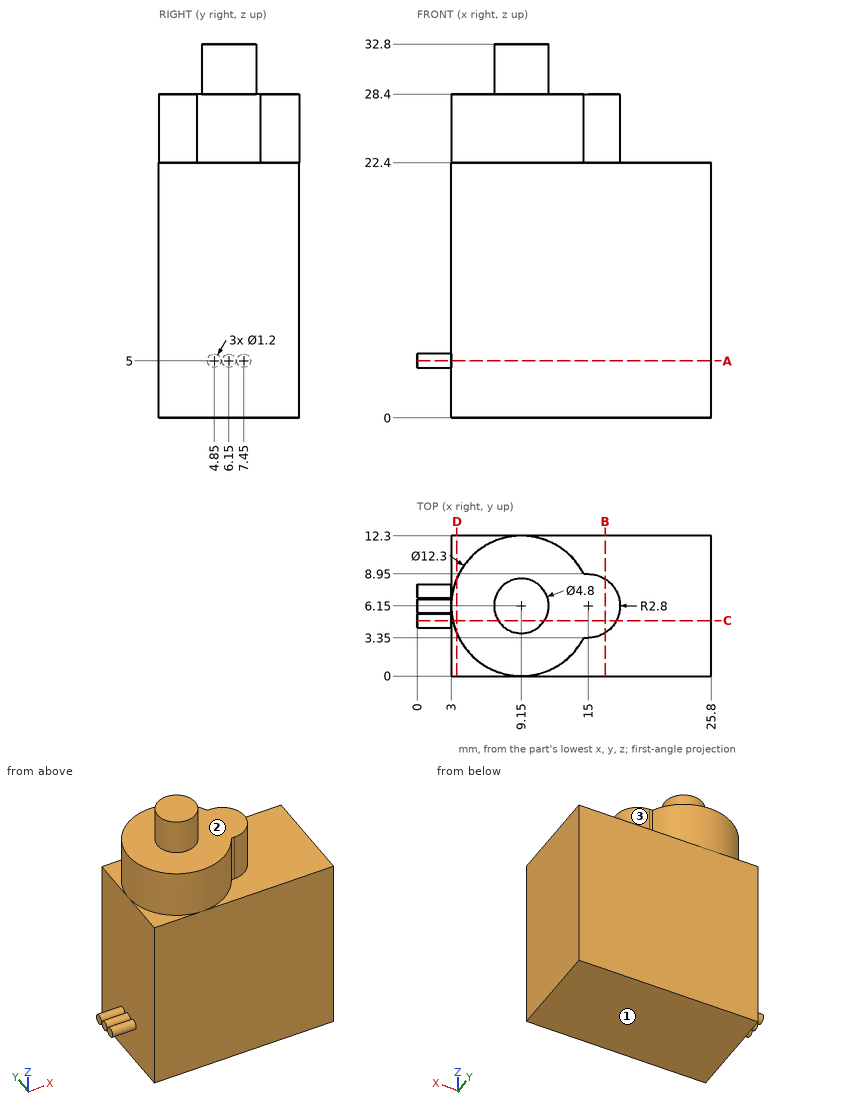
Answer from the drawing. Dimensions are ordinates in mm from the lowest x, y and z of the part. A direction names the side the tool comes from. Give positions to 0.01 mm unless a question says otherwise; leave off trailing zeros. Write each loop counter-clockwise with the first axis right and the second up, starting at its lowest first coordinate (ties: lowest second). Pieces come first, ordered by that corner, then holes.
1) A tool of negligible diameter and unlimited length cuts with its end or side. For the marked faces 1, 2 and 3, from which of +Z, -Z, +X, -X, +Y, -Y can it reach the whole face along a straight path? Write none if from no direction.
2) Given P1, Ø3, axis at x = 5, y = 10, coming from the +Z side; P2, Ø5, axis at y = 8.5, z = 29, coming from the +X side; P3, Ø6, axis at y = 7.5, z = 11.5, coming from the -X side, each flat-ended and moving along its own axis, determine where each tip first touches the part or whether it passes through.
3) Section D-D (x = 3.5) is taken. Write down the section's boundary in (y, z), and give its area (3 significant figures).
4) Section C-C (y = 4.85) is taken. Write down the section's boundary in (x, z), and give its area (3 significant figures).
5) Section B-B (x = 16.5) is taken. Write down the section's boundary in (y, z), and give its area (3 significant figures).
6) Find the intervals of material crossed by L1, parallel to X at y = 1.5, z = 17; L2, parallel to Z at x = 21.75, y = 9.5; L3, parallel to Z at x = 16, y = 5.5, in increasing order.
7) Section A-A (z = 5) is taken. Write down the section's boundary in (x, y).
Response:
1. face 1: -Z, +X, -X, +Y, -Y
1. face 2: +Z
1. face 3: +Z, +X
2. P1: stops at z = 28.4
2. P2: stops at x = 17.8
2. P3: stops at x = 3
3. outline: (0, 0) - (12.3, 0) - (12.3, 22.4) - (8.58, 22.4) - (8.58, 28.4) - (3.72, 28.4) - (3.72, 22.4) - (0, 22.4) - close
3. area: 305 mm2
4. outline: (0, 4.4) - (3, 4.4) - (3, 0) - (25.8, 0) - (25.8, 22.4) - (17.48, 22.4) - (17.48, 28.4) - (11.17, 28.4) - (11.17, 32.8) - (7.13, 32.8) - (7.13, 28.4) - (3.14, 28.4) - (3.14, 22.4) - (3, 22.4) - (3, 5.6) - (0, 5.6) - close
4. area: 618 mm2
5. outline: (0, 0) - (12.3, 0) - (12.3, 22.4) - (8.51, 22.4) - (8.51, 28.4) - (3.79, 28.4) - (3.79, 22.4) - (0, 22.4) - close
5. area: 304 mm2
6. L1: x = 3 to 25.8
6. L2: z = 0 to 22.4
6. L3: z = 0 to 28.4
7. outline: (0, 4.25) - (3, 4.25) - (3, 0) - (25.8, 0) - (25.8, 12.3) - (3, 12.3) - (3, 8.05) - (0, 8.05) - (0, 6.85) - (3, 6.85) - (3, 6.75) - (0, 6.75) - (0, 5.55) - (3, 5.55) - (3, 5.45) - (0, 5.45) - close
